```python
from build123d import *

# Parameters (mm, degrees)
BOSS_EXTRU_1_DEPTH = 15
CONG_1_R           = 0.5


with BuildPart() as part:
    # Esquisse1 → Boss.-Extru.1 (new body)
    with BuildSketch(Plane.XY):
        with BuildLine():
            Line((8.084553173, 6.7), (18.084553173, 6.7))
            ThreePointArc((18.084553173, 6.7), (24.784553173, 0), (18.084553173, -6.7))
            Line((18.084553173, -6.7), (8.084553173, -6.7))
            ThreePointArc((8.084553173, -6.7), (-0.157024945, -10.498825799), (-8.281308366, -6.45522515))
            Line((-8.281308366, -6.45522515), (-12.931761957, -8.291874654))
            ThreePointArc((-12.931761957, -8.291874654), (-7.243702669, -15.843181093), (2.093196436, -17.325936129))
            Line((2.093196436, -17.325936129), (18.084553173, -13.642820952))
            ThreePointArc((18.084553173, -13.642820952), (28.942350685, 0), (18.084553173, 13.642820952))
            Line((18.084553173, 13.642820952), (2.093196436, 17.325936129))
            ThreePointArc((2.093196436, 17.325936129), (-7.243702669, 15.843181093), (-12.931761957, 8.291874654))
            Line((-12.931761957, 8.291874654), (-8.281308366, 6.45522515))
            ThreePointArc((-8.281308366, 6.45522515), (-0.157024945, 10.498825799), (8.084553173, 6.7))
        make_face()
    extrude(amount=BOSS_EXTRU_1_DEPTH)

    # Congé1
    cong_1_edges = [part.edges().sort_by_distance(p)[0] for p in [
        (24.784553173, 0, 15),
        (24.784553173, 0, 0),
        (13.084553173, 6.7, 15),
        (13.084553173, 6.7, 0),
        (-10.606535162, 7.373549902, 15),
        (-10.606535162, 7.373549902, 0),
        (-8.281308366, 6.45522515, 7.5),
        (-0.157024945, 10.498825799, 15),
        (8.084553173, 6.7, 7.5),
        (-0.157024945, 10.498825799, 0),
        (13.084553173, -6.7, 15),
        (13.084553173, -6.7, 0),
        (-12.931761957, 8.291874654, 7.5),
    ]]
    fillet(cong_1_edges, radius=CONG_1_R)


solid = part.part
```
For this review, take the finished solid that the model builds, in its own axes (mm). A direction names the side the tool comes from. Coordinates: 2 decimals unless noted, no trailing zeros. Write each loop counter-clockwise with the first axis right and the second up, starting at its lowest first coordinate (ties: lowest second). Pieces come first, ordered by that corner, then holes. Notation, with made-up numbers: (-14.5, -17) - (6.5, -17) arc R10 ccw to (6.5, 0) - close; hole circle Ø8 at (77, -21). An arc over 180 degrees is marked (long way). Answer in a Markdown table with one row per item. Add a question column.
Q1. We need section C-C, the plane y = 0. State the section outline as (x, z) points, and give its area (3 significant figures).
Q2. For P1, Ø5, axis at x = 14, z = 6.5, coming from the +Y side; P2, Ø8, axis at x = 14.5, z = 13, coming from the +Y side; P3, Ø3, axis at x = 11.5, z = 7, coming from the -Y side; P4, Ø6, axis at x = 0, y = -6, coming from the -Z side, all flat-tipped, find the tip position at first contact; note any pin that passes through.
Q3. Draft analysis for pull direction Y (two halves, no side actions). For faces 1 (the flat face through (8, -8, 0)), 2 (the cylindrical face through (-7.36, -15.773, 7.395)), 3 (the cylindrical face through (-0.2, 10.5, 7.4)), 4 (the cylindrical face through (-6.929, 16.026, 7.395)), state which applies: +Y half, -Y half, draft (parallel to the pull), parting line (faces both ways), or undercut.
Q4. Tool access review of faces 5 (the cylindrical face through (0, -10.5, 7.4)), 6 (the cylindrical face through (-10.72, 7.57, 14.85)), 7 (the cylindrical face through (-10.72, 7.57, 0.15)), 8 (the flat face through (10.2, 15.46, 7.4)), 9 (the flat face through (-10.593, 7.368, 7.402)): name each direction out of +Z, -Z, +X, -X, +Y, -Y from which nothing blocks a thin tool from reaching the whole face with its end or side.
Q5. For probe 1 along Y at (x, z) = (-7, 1.75); probe 2 along Y at (x, z) = (23, 6.5); probe 3 along X at (y, z) = (9.5, 2.5), list the stretches that pass through material, from the lowest coordinate up.
Q6. We need section A-A, the plane z = 7.25. State the section outline as (x, y) points.
Q7. We need section B-B, the plane x = 9. State the section outline as (y, z) points, and give its area (3 significant figures).
Answer list:
| question | item | result |
|---|---|---|
| 1 | outline | (24.78, 0.5) arc R0.5 ccw to (25.28, 0) - (28.94, 0) - (28.94, 15) - (25.28, 15) arc R0.5 ccw to (24.78, 14.5) - close |
| 1 | area | 62.3 mm2 |
| 2 | P1 | stops at y = 15.16 |
| 2 | P2 | stops at y = 15.39 |
| 2 | P3 | stops at y = -15.5 |
| 2 | P4 | passes through |
| 3 | face 1 | draft |
| 3 | face 2 | -Y half |
| 3 | face 3 | undercut |
| 3 | face 4 | +Y half |
| 4 | face 5 | +Z, -Z |
| 4 | face 6 | +Z, -X |
| 4 | face 7 | -Z, -X |
| 4 | face 8 | +Z, -Z, +X, +Y |
| 4 | face 9 | +Z, -Z, -X |
| 5 | probe 1 | y = -15.99 to -7.83, 7.83 to 15.99 |
| 5 | probe 2 | y = -11.45 to -4.55, 4.55 to 11.45 |
| 5 | probe 3 | x = -12.54 to -4.47, 4.47 to 25.23 |
| 6 | outline | (-12.93, -8.29) arc R12.62 ccw to (2.09, -17.33) - (18.08, -13.64) arc R14 ccw to (18.08, 13.64) - (2.09, 17.33) arc R12.62 ccw to (-12.8, 8.74) arc R0.5 ccw to (-12.51, 8.13) - (-8.62, 6.59) arc R0.5 ccw to (-8.06, 6.73) arc R10.5 cw to (7.94, 6.87) arc R0.5 ccw to (8.32, 6.7) - (18.08, 6.7) arc R6.7 cw to (18.08, -6.7) - (8.08, -6.7) arc R10.5 cw to (-8.28, -6.46) - close |
| 7 | outline | (-15.74, 0) - (-7.2, 0) arc R0.5 ccw to (-6.7, 0.5) - (-6.7, 14.5) arc R0.5 ccw to (-7.2, 15) - (-15.74, 15) - close; (6.7, 0.5) arc R0.5 ccw to (7.2, 0) - (15.74, 0) - (15.74, 15) - (7.2, 15) arc R0.5 ccw to (6.7, 14.5) - close |
| 7 | area | 271 mm2 |
